```python
from build123d import *

# Parameters (mm, degrees)
BASE_FLANGE1_DEPTH       = 80
CUT_EXTRUDE1_START       = 48.39544582
CUT_EXTRUDE1_OUTLINE_W   = 3
CUT_EXTRUDE1_OUTLINE_H   = 13
CUT_EXTRUDE1_DEPTH       = 24
CUT_EXTRUDE1_START_2     = -46.394569282
CUT_EXTRUDE1_2_OUTLINE_R = 1
CUT_EXTRUDE1_2_DEPTH     = 46.394569282


# Read off the part's stored shape, not the designer's step: Cut-Extrude1
# Sheet-metal steps are written as plain solids
with BuildPart() as part:
    # Sketch1 → Base-Flange1 (new body)
    with BuildSketch(Plane.XY):
        with BuildLine():
            Line((23.197284641, 47.603861413), (23.197284641, 18.763363208))
            ThreePointArc((23.197284641, 18.763363208), (21.732818547, 15.227829302), (18.197284641, 13.763363208))
            Line((18.197284641, 13.763363208), (-18.197284641, 13.763363208))
            ThreePointArc((-18.197284641, 13.763363208), (-21.732818547, 15.227829302), (-23.197284641, 18.763363208))
            Line((-23.197284641, 18.763363208), (-23.197284641, 47.603861413))
            Line((-23.197284641, 47.603861413), (-20.197284641, 47.603861413))
            Line((-20.197284641, 47.603861413), (-20.197284641, 18.763363208))
            ThreePointArc((-20.197284641, 18.763363208), (-19.611498203, 17.349149646), (-18.197284641, 16.763363208))
            Line((-18.197284641, 16.763363208), (18.197284641, 16.763363208))
            ThreePointArc((18.197284641, 16.763363208), (19.611498203, 17.349149646), (20.197284641, 18.763363208))
            Line((20.197284641, 18.763363208), (20.197284641, 47.603861413))
            Line((20.197284641, 47.603861413), (23.197284641, 47.603861413))
        make_face()
    extrude(amount=BASE_FLANGE1_DEPTH)

    # Cut-Extrude1 outline → Cut-Extrude1 (cut)
    with BuildSketch(Plane.XY.offset(CUT_EXTRUDE1_START)):
        with BuildLine():
            Line((-20.197284641, 18.763363208), (-20.197284641, 31.428624583))
            Line((-20.197284641, 31.428624583), (-23.197284641, 31.428624583))
            Line((-23.197284641, 31.428624583), (-23.197284641, 18.763363208))
            ThreePointArc((-23.197284641, 18.763363208), (-23.17962128, 18.343456534), (-23.126755995, 17.926516645))
            Line((-23.126755995, 17.926516645), (-20.169073182, 18.428624583))
            ThreePointArc((-20.169073182, 18.428624583), (-20.190219297, 18.595400538), (-20.197284641, 18.763363208))
        make_face()
        with Locations((-21.697284641, 38.186330489)):
            Rectangle(CUT_EXTRUDE1_OUTLINE_W, CUT_EXTRUDE1_OUTLINE_H)
        with BuildLine():
            Line((23.197284641, 18.763363208), (23.197284641, 31.428624583))
            Line((23.197284641, 31.428624583), (20.197284641, 31.428624583))
            Line((20.197284641, 31.428624583), (20.197284641, 18.763363208))
            ThreePointArc((20.197284641, 18.763363208), (20.190219297, 18.595400538), (20.169073182, 18.428624583))
            Line((20.169073182, 18.428624583), (23.126755995, 17.926516645))
            ThreePointArc((23.126755995, 17.926516645), (23.17962128, 18.343456534), (23.197284641, 18.763363208))
        make_face()
        with Locations((21.697284641, 38.186330489)):
            Rectangle(CUT_EXTRUDE1_OUTLINE_W, CUT_EXTRUDE1_OUTLINE_H)
    extrude(amount=CUT_EXTRUDE1_DEPTH, mode=Mode.SUBTRACT)

    # Cut-Extrude1 2 outline → Cut-Extrude1 2 (cut)
    with BuildSketch(Plane.ZY.offset(23.197284641).offset(CUT_EXTRUDE1_START_2)):
        with Locations((74.29544582, 24.928624583)):
            Circle(CUT_EXTRUDE1_2_OUTLINE_R)
        with Locations((46.49544582, 24.928624583)):
            Circle(CUT_EXTRUDE1_2_OUTLINE_R)
        with Locations((74.29544582, 38.186330489)):
            Circle(CUT_EXTRUDE1_2_OUTLINE_R)
        with Locations((46.49544582, 38.186330489)):
            Circle(CUT_EXTRUDE1_2_OUTLINE_R)
    extrude(amount=CUT_EXTRUDE1_2_DEPTH, mode=Mode.SUBTRACT)


solid = part.part
```
Input: part model. Units: mm. Frame: model coordinates. A direction names the side the tool comes from. Give positions to 0.01 mm unless a question says otherwise; leave off trailing zeros. Order: outer loops, then holes, each group sorted by start corner. A loop starts at its lowest first (then second) coordinate and runs counter-clockwise, first axis right, second up. Notation, with made-up numbers: M 53.5,39.5 L 111.5,39.5 A9 cw 111.5,45.5 Z; hole C -4.5,74.5 d7. An arc over 180 degrees is marked long. Return JSON: item names as keys, results as strings.
Item 1: First-contact query: P1, Ø2.5, axis at x = -21, z = 54.5, coming from the -Y side; P2, Ø2, axis at x = -5.5, z = 45.5, coming from the +Y side; P3, Ø10, axis at x = 14.5, z = 67, coming from the +Y side. Flat tips, straight axial feed; report the tip coordinate or a pass-through.
Solutions:
{"P1": "y = 14.01", "P2": "y = 16.76", "P3": "y = 17.25"}
Item 2: Access query for faces 1 (the flat face through (0, 16, 80)), 2 (the flat face through (22, 38, 48.395)), 3 (the flat face through (-21.669, 18.174, 60.227)). Directions: +Z, -Z, +X, -X, +Y, -Y. A direction counts if a zero-diameter tool reaches every point of the face in a straight line with its end or side. Return the directions, or none.
Solutions:
{"face 1": "+Z, +X, -X, +Y, -Y", "face 2": "+X, -X", "face 3": "-X"}
Item 3: Cut plane C-C (y = 45.5). Return loops of the section in (x, z), then the cut area to 3 significant figures.
Solutions:
{"outline": "M -23.2,0 L -20.2,0 L -20.2,80 L -23.2,80 Z; M 20.2,0 L 23.2,0 L 23.2,80 L 20.2,80 Z", "area": "480 mm^2"}
Item 4: Cut plane A-A (z = 69.5). Return loops of the section in (x, y), then the cut area to 3 significant figures.
Solutions:
{"outline": "M -23.2,31.43 L -20.2,31.43 L -20.2,31.69 L -23.2,31.69 Z; M -23.2,44.69 L -20.2,44.69 L -20.2,47.6 L -23.2,47.6 Z; M -23.13,17.93 A5 ccw -18.2,13.76 L 18.2,13.76 A5 ccw 23.13,17.93 L 20.17,18.43 A2 cw 18.2,16.76 L -18.2,16.76 A2 cw -20.17,18.43 Z; M 20.2,31.43 L 23.2,31.43 L 23.2,31.69 L 20.2,31.69 Z; M 20.2,44.69 L 23.2,44.69 L 23.2,47.6 L 20.2,47.6 Z", "area": "158 mm^2"}
Item 5: Cut plane B-B (y = 35.5). Return loops of the section in (x, z).
Solutions:
{"outline": "M -23.2,0 L -20.2,0 L -20.2,48.4 L -23.2,48.4 Z; M -23.2,72.4 L -20.2,72.4 L -20.2,80 L -23.2,80 Z; M 20.2,0 L 23.2,0 L 23.2,48.4 L 20.2,48.4 Z; M 20.2,72.4 L 23.2,72.4 L 23.2,80 L 20.2,80 Z"}
Item 6: Cut plane D-D (z = 5.5). Return loops of the section in (x, y), then the cut area to 3 significant figures.
Solutions:
{"outline": "M -23.2,18.76 A5 ccw -18.2,13.76 L 18.2,13.76 A5 ccw 23.2,18.76 L 23.2,47.6 L 20.2,47.6 L 20.2,18.76 A2 cw 18.2,16.76 L -18.2,16.76 A2 cw -20.2,18.76 L -20.2,47.6 L -23.2,47.6 Z", "area": "315 mm^2"}
Item 7: Pull-direction query (X, two-part tool) for faces 4 (the flat face through (22, 44.686, 60)), 5 (the flat face through (-23.197, 33, 31)), 6 (the flat face through (20.197, 33, 31)); classes: +X half, -X half, draft (parallel to the pull), parting line (faces both ways), or undercut.
Solutions:
{"face 4": "draft", "face 5": "-X half", "face 6": "undercut"}
Item 8: Ray query, probe 1 along X at (y, z) = (41.5, 75); probe 2 along Y at (x, z) = (7.5, 35.5); probe 3 along X at (y, z) = (17, 63.5). Return the intervals inside material, ascending.
Solutions:
{"probe 1": "-23.2 to -20.2, 20.2 to 23.2", "probe 2": "13.76 to 16.76", "probe 3": "-22.88 to -19.14, 19.14 to 22.88"}
